Can you work these out from the model? Positions are in its coordinate system, mm. Face numbers are marked on the shaded views. A direction names the side the tool comes from. Give positions to 0.01 mm unless a question says otherwise; leave off trailing zeros. Loops run counter-clockwise (first coordinate to the right, second up) from the corner with the lowest first, then second, coordinate; pieces in that order, holes last. Notation, with made-up numbers: (63, 27.25) - (76, 27.25) arc R34 ccw to (76, 63.25) - close; hole circle Ø8 at (3, 13). An arc over 180 degrees is marked (long way). Answer as a JSON object with one key per item and string values.
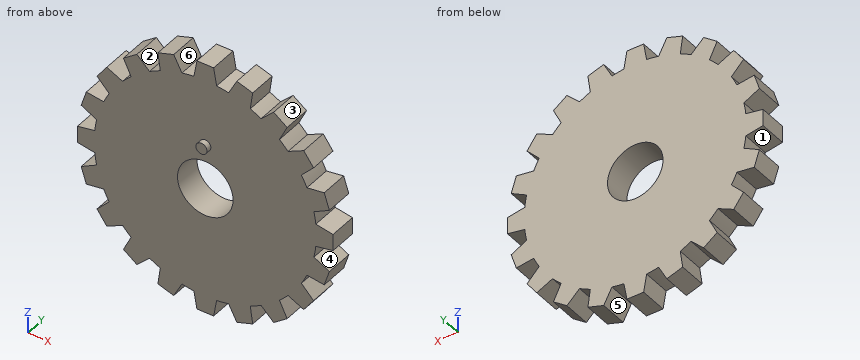
```python
from build123d import *

# Parameters (mm, degrees)
F0_R     = 5
F1_DEPTH = 5
F2_R     = 1
F3_DEPTH = 1


with BuildPart() as f1:
    # F0 (on Front) → F1 (new body)
    with BuildSketch(Plane.XZ):
        with BuildLine():
            ThreePointArc((19.894917, -2.04751), (19.973712, -1.025102), (20, 0))
            ThreePointArc((20, 0), (19.973712, 1.025102), (19.894917, 2.04751))
            ThreePointArc((19.894917, 2.04751), (19.753767, 3.128689), (19.553905, 4.20057))
            ThreePointArc((19.553905, 4.20057), (19.02113, 6.18034), (18.288475, 8.095165))
            ThreePointArc((18.288475, 8.095165), (17.82013, 9.07981), (17.298822, 10.037468))
            ThreePointArc((17.298822, 10.037468), (16.18034, 11.755705), (14.891829, 13.350409))
            ThreePointArc((14.891829, 13.350409), (14.142136, 14.142136), (13.350409, 14.891829))
            ThreePointArc((13.350409, 14.891829), (11.755705, 16.18034), (10.037468, 17.298822))
            ThreePointArc((10.037468, 17.298822), (9.07981, 17.82013), (8.095165, 18.288475))
            ThreePointArc((8.095165, 18.288475), (6.18034, 19.02113), (4.20057, 19.553905))
            ThreePointArc((4.20057, 19.553905), (3.128689, 19.753767), (2.04751, 19.894917))
            ThreePointArc((2.04751, 19.894917), (0, 20), (-2.04751, 19.894917))
            ThreePointArc((-2.04751, 19.894917), (-3.128689, 19.753767), (-4.20057, 19.553905))
            ThreePointArc((-4.20057, 19.553905), (-6.18034, 19.02113), (-8.095165, 18.288475))
            ThreePointArc((-8.095165, 18.288475), (-9.07981, 17.82013), (-10.037468, 17.298822))
            ThreePointArc((-10.037468, 17.298822), (-11.755705, 16.18034), (-13.350409, 14.891829))
            ThreePointArc((-13.350409, 14.891829), (-14.142136, 14.142136), (-14.891829, 13.350409))
            ThreePointArc((-14.891829, 13.350409), (-16.18034, 11.755705), (-17.298822, 10.037468))
            ThreePointArc((-17.298822, 10.037468), (-17.82013, 9.07981), (-18.288475, 8.095165))
            ThreePointArc((-18.288475, 8.095165), (-19.02113, 6.18034), (-19.553905, 4.20057))
            ThreePointArc((-19.553905, 4.20057), (-19.753767, 3.128689), (-19.894917, 2.04751))
            ThreePointArc((-19.894917, 2.04751), (-20, 0), (-19.894917, -2.04751))
            ThreePointArc((-19.894917, -2.04751), (-19.753767, -3.128689), (-19.553905, -4.20057))
            ThreePointArc((-19.553905, -4.20057), (-19.02113, -6.18034), (-18.288475, -8.095165))
            ThreePointArc((-18.288475, -8.095165), (-17.82013, -9.07981), (-17.298822, -10.037468))
            ThreePointArc((-17.298822, -10.037468), (-16.18034, -11.755705), (-14.891829, -13.350409))
            ThreePointArc((-14.891829, -13.350409), (-14.142136, -14.142136), (-13.350409, -14.891829))
            ThreePointArc((-13.350409, -14.891829), (-11.755705, -16.18034), (-10.037468, -17.298822))
            ThreePointArc((-10.037468, -17.298822), (-9.07981, -17.82013), (-8.095165, -18.288475))
            ThreePointArc((-8.095165, -18.288475), (-6.18034, -19.02113), (-4.20057, -19.553905))
            ThreePointArc((-4.20057, -19.553905), (-3.128689, -19.753767), (-2.04751, -19.894917))
            ThreePointArc((-2.04751, -19.894917), (0, -20), (2.04751, -19.894917))
            ThreePointArc((2.04751, -19.894917), (3.128689, -19.753767), (4.20057, -19.553905))
            ThreePointArc((4.20057, -19.553905), (6.18034, -19.02113), (8.095165, -18.288475))
            ThreePointArc((8.095165, -18.288475), (9.07981, -17.82013), (10.037468, -17.298822))
            ThreePointArc((10.037468, -17.298822), (11.755705, -16.18034), (13.350409, -14.891829))
            ThreePointArc((13.350409, -14.891829), (14.142136, -14.142136), (14.891829, -13.350409))
            ThreePointArc((14.891829, -13.350409), (16.18034, -11.755705), (17.298822, -10.037468))
            ThreePointArc((17.298822, -10.037468), (17.82013, -9.07981), (18.288475, -8.095165))
            ThreePointArc((18.288475, -8.095165), (19.02113, -6.18034), (19.553905, -4.20057))
            ThreePointArc((19.553905, -4.20057), (19.753767, -3.128689), (19.894917, -2.04751))
        make_face()
        Circle(F0_R, mode=Mode.SUBTRACT)
        with BuildLine():
            ThreePointArc((19.894917, 2.04751), (19.973712, 1.025102), (20, 0))
            ThreePointArc((20, 0), (19.973712, -1.025102), (19.894917, -2.04751))
            Line((19.894917, -2.04751), (23, -1.5))
            Line((23, -1.5), (23, 1.5))
            Line((23, 1.5), (19.894917, 2.04751))
        make_face()
        with BuildLine():
            ThreePointArc((18.288475, 8.095165), (19.02113, 6.18034), (19.553905, 4.20057))
            Line((19.553905, 4.20057), (22.337825, 5.680806))
            Line((22.337825, 5.680806), (21.410774, 8.533976))
            Line((21.410774, 8.533976), (18.288475, 8.095165))
        make_face()
        with BuildLine():
            Line((22.337825, -5.680806), (19.553905, -4.20057))
            ThreePointArc((19.553905, -4.20057), (19.02113, -6.18034), (18.288475, -8.095165))
            Line((18.288475, -8.095165), (21.410774, -8.533976))
            Line((21.410774, -8.533976), (22.337825, -5.680806))
        make_face()
        with BuildLine():
            ThreePointArc((14.891829, 13.350409), (16.18034, 11.755705), (17.298822, 10.037468))
            Line((17.298822, 10.037468), (19.489069, 12.305535))
            Line((19.489069, 12.305535), (17.725713, 14.732586))
            Line((17.725713, 14.732586), (14.891829, 13.350409))
        make_face()
        with BuildLine():
            Line((19.489069, -12.305535), (17.298822, -10.037468))
            ThreePointArc((17.298822, -10.037468), (16.18034, -11.755705), (14.891829, -13.350409))
            Line((14.891829, -13.350409), (17.725713, -14.732586))
            Line((17.725713, -14.732586), (19.489069, -12.305535))
        make_face()
        with BuildLine():
            ThreePointArc((10.037468, 17.298822), (11.755705, 16.18034), (13.350409, 14.891829))
            Line((13.350409, 14.891829), (14.732586, 17.725713))
            Line((14.732586, 17.725713), (12.305535, 19.489069))
            Line((12.305535, 19.489069), (10.037468, 17.298822))
        make_face()
        with BuildLine():
            Line((14.732586, -17.725713), (13.350409, -14.891829))
            ThreePointArc((13.350409, -14.891829), (11.755705, -16.18034), (10.037468, -17.298822))
            Line((10.037468, -17.298822), (12.305535, -19.489069))
            Line((12.305535, -19.489069), (14.732586, -17.725713))
        make_face()
        with BuildLine():
            ThreePointArc((4.20057, 19.553905), (6.18034, 19.02113), (8.095165, 18.288475))
            Line((8.095165, 18.288475), (8.533976, 21.410774))
            Line((8.533976, 21.410774), (5.680806, 22.337825))
            Line((5.680806, 22.337825), (4.20057, 19.553905))
        make_face()
        with BuildLine():
            Line((8.533976, -21.410774), (8.095165, -18.288475))
            ThreePointArc((8.095165, -18.288475), (6.18034, -19.02113), (4.20057, -19.553905))
            Line((4.20057, -19.553905), (5.680806, -22.337825))
            Line((5.680806, -22.337825), (8.533976, -21.410774))
        make_face()
        with BuildLine():
            ThreePointArc((-2.04751, 19.894917), (0, 20), (2.04751, 19.894917))
            Line((2.04751, 19.894917), (1.5, 23))
            Line((1.5, 23), (-1.5, 23))
            Line((-1.5, 23), (-2.04751, 19.894917))
        make_face()
        with BuildLine():
            Line((1.5, -23), (2.04751, -19.894917))
            ThreePointArc((2.04751, -19.894917), (0, -20), (-2.04751, -19.894917))
            Line((-2.04751, -19.894917), (-1.5, -23))
            Line((-1.5, -23), (1.5, -23))
        make_face()
        with BuildLine():
            ThreePointArc((-8.095165, 18.288475), (-6.18034, 19.02113), (-4.20057, 19.553905))
            Line((-4.20057, 19.553905), (-5.680806, 22.337825))
            Line((-5.680806, 22.337825), (-8.533976, 21.410774))
            Line((-8.533976, 21.410774), (-8.095165, 18.288475))
        make_face()
        with BuildLine():
            Line((-5.680806, -22.337825), (-4.20057, -19.553905))
            ThreePointArc((-4.20057, -19.553905), (-6.18034, -19.02113), (-8.095165, -18.288475))
            Line((-8.095165, -18.288475), (-8.533976, -21.410774))
            Line((-8.533976, -21.410774), (-5.680806, -22.337825))
        make_face()
        with BuildLine():
            ThreePointArc((-13.350409, 14.891829), (-11.755705, 16.18034), (-10.037468, 17.298822))
            Line((-10.037468, 17.298822), (-12.305535, 19.489069))
            Line((-12.305535, 19.489069), (-14.732586, 17.725713))
            Line((-14.732586, 17.725713), (-13.350409, 14.891829))
        make_face()
        with BuildLine():
            Line((-12.305535, -19.489069), (-10.037468, -17.298822))
            ThreePointArc((-10.037468, -17.298822), (-11.755705, -16.18034), (-13.350409, -14.891829))
            Line((-13.350409, -14.891829), (-14.732586, -17.725713))
            Line((-14.732586, -17.725713), (-12.305535, -19.489069))
        make_face()
        with BuildLine():
            ThreePointArc((-17.298822, 10.037468), (-16.18034, 11.755705), (-14.891829, 13.350409))
            Line((-14.891829, 13.350409), (-17.725713, 14.732586))
            Line((-17.725713, 14.732586), (-19.489069, 12.305535))
            Line((-19.489069, 12.305535), (-17.298822, 10.037468))
        make_face()
        with BuildLine():
            Line((-17.725713, -14.732586), (-14.891829, -13.350409))
            ThreePointArc((-14.891829, -13.350409), (-16.18034, -11.755705), (-17.298822, -10.037468))
            Line((-17.298822, -10.037468), (-19.489069, -12.305535))
            Line((-19.489069, -12.305535), (-17.725713, -14.732586))
        make_face()
        with BuildLine():
            ThreePointArc((-19.553905, 4.20057), (-19.02113, 6.18034), (-18.288475, 8.095165))
            Line((-18.288475, 8.095165), (-21.410774, 8.533976))
            Line((-21.410774, 8.533976), (-22.337825, 5.680806))
            Line((-22.337825, 5.680806), (-19.553905, 4.20057))
        make_face()
        with BuildLine():
            Line((-21.410774, -8.533976), (-18.288475, -8.095165))
            ThreePointArc((-18.288475, -8.095165), (-19.02113, -6.18034), (-19.553905, -4.20057))
            Line((-19.553905, -4.20057), (-22.337825, -5.680806))
            Line((-22.337825, -5.680806), (-21.410774, -8.533976))
        make_face()
        with BuildLine():
            ThreePointArc((-19.894917, -2.04751), (-20, 0), (-19.894917, 2.04751))
            Line((-19.894917, 2.04751), (-23, 1.5))
            Line((-23, 1.5), (-23, -1.5))
            Line((-23, -1.5), (-19.894917, -2.04751))
        make_face()
    extrude(amount=F1_DEPTH)

    # F2 (on face) → F3 (join)
    with BuildSketch(Plane.XZ.offset(5)):
        with Locations((0, 8)):
            Circle(F2_R)
    extrude(amount=F3_DEPTH)


solid = f1.part
```
1) Imagine slicing it at A-A on z = 0. Write out the boundary of the cut face in (x, y).
Check sheet entries:
{"outline": "(-23, -5) - (-5, -5) - (-5, 0) - (-23, 0) - close; (5, -5) - (23, -5) - (23, 0) - (5, 0) - close"}
2) I need wall thicknesses on L1, parallel to Z at x = 0, y = -2.25; L2, parallel to X at y = -2.4, z = -18; L3, parallel to Y at x = 6.5, z = -4. Which ranges of each line are inside material? Lowest first, please.
Check sheet entries:
{"L1": "-23 to -5, 5 to 23", "L2": "-14.36 to -10.76, -8.72 to 8.72, 10.76 to 14.36", "L3": "-5 to 0"}
3) If we mould it in two halves opening along X, with no side actions, what happens to the marked faces 1, 2 and 3? For each: released by +X, released by -X, zero draft, split by the parting line, or undercut.
Check sheet entries:
{"face 1": "released by -X", "face 2": "undercut", "face 3": "released by +X"}
4) I'm going to push flat-ended pins straight in: P1, Ø12, axis at x = -18, z = 12, coming from the -Y side; P2, Ø1.5, axis at x = 17.5, y = -4.5, coming from the -Z side; P3, Ø3, axis at y = -5.5, z = 10.5, coming from the -X side. Where does each tip first touch, or does it pass through?
Check sheet entries:
{"P1": "y = -5", "P2": "z = -14.73", "P3": "x = -19.11"}
5) Which directions (+Z, -Z, +X, -X, +Y, -Y) give clear straight access to the entire face, cutting with the end or side of a thin tool? Please do the marked faces 4, 5 and 6.
Check sheet entries:
{"face 4": "+X, +Y, -Y", "face 5": "-Z, +Y, -Y", "face 6": "+Z, +Y, -Y"}
6) Imagine slicing it at C-C on x = -6.5. Write out the boundary of the cut face in (y, z).
Check sheet entries:
{"outline": "(-5, -22.07) - (0, -22.07) - (0, 22.07) - (-5, 22.07) - close"}
7) Imagine slicing it at B-B on x = 0. Write out the boundary of the cut face in (y, z), and give its area (3 significant figures).
Check sheet entries:
{"outline": "(-6, 7) - (-5, 7) - (-5, 5) - (0, 5) - (0, 23) - (-5, 23) - (-5, 9) - (-6, 9) - close; (-5, -23) - (0, -23) - (0, -5) - (-5, -5) - close", "area": "182 mm2"}
